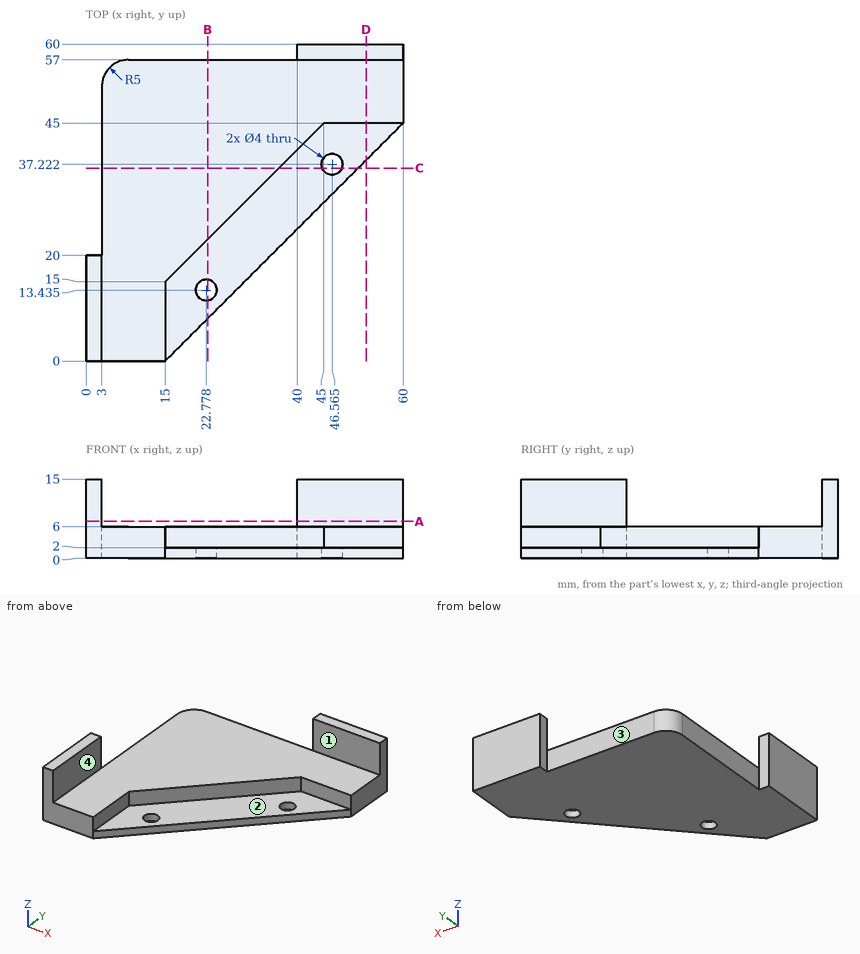
For this review, use the dimensioned drawing (mm, ordinates from the lowest corner) and the shaded views. A direction names the side the tool comes from. Round coordinates to 2 decimals unless told otherwise and drop trailing zeros. Order: outer loops, then holes, each group sorted by start corner. A loop starts at its lowest first (then second) coordinate and runs counter-clockwise, first axis right, second up. Notation, with made-up numbers: (72.5, 56.25) -> (77.5, 56.25) arc R20 ccw to (77.5, 93.25) -> close; hole circle Ø6 at (48, -19.75). An arc over 180 degrees is marked (long way). One line per item, written item: value. Start each with the question number.
Q1. Take a section at C-C (y = 36.5). Write out the cut boundary in (x, z), and give its area (3 significant figures).
Q2. Wall thickness on line 1 (Z direction, x = 14, y = 33); line 2 (Y direction, x = 55, z = 1.5); line 3 (Z direction, x = 17.5, y = 8.5): over which ranges is each line inside the solid? List them lowest first.
Q3. Take a section at D-D (x = 53). Write out the cut boundary in (y, z).
Q4. Clearance check with flat-ended pins moving along their axes: pin 1 Ø10 at (x, y) = (13.5, 27.5) entering from +Z; pin 2 Ø1.8 at (x, z) = (23.5, 2) entering from +Y; pin 3 Ø6.5 at (x, y) = (46.56, 37.22) entering from +Z; pin 4 Ø5 at (y, z) = (28.5, 10) entering from -X. State where each tip first meets the part, or that it passes through.
Q5. Take a section at A-A (z = 7). Write out the cut boundary in (x, y).
Q6. Take a section at B-B (x = 23). Write out the cut boundary in (y, z).
Q7. Machinability: for the marked faces 1, 2, 3 and 4, which of the approach directions +Z, -Z, +X, -X, +Y, -Y give a long, thin tool a straight path to every point of the face, cutting with its end or side? Answer none if there is none.
Reported:
1. outline: (3, 0) -> (44.7, 0) -> (44.7, 2) -> (36.5, 2) -> (36.5, 6) -> (3, 6) -> close; (48.43, 0) -> (51.5, 0) -> (51.5, 2) -> (48.43, 2) -> close
1. area: 224 mm2
2. line 1: z = 0 to 6
2. line 2: y = 40 to 60
2. line 3: z = 0 to 2
3. outline: (38, 0) -> (60, 0) -> (60, 15) -> (57, 15) -> (57, 6) -> (45, 6) -> (45, 2) -> (38, 2) -> close
4. pin 1: stops at z = 6
4. pin 2: stops at y = 57
4. pin 3: stops at z = 2
4. pin 4: passes through
5. outline: (0, 0) -> (3, 0) -> (3, 20) -> (0, 20) -> close; (40, 57) -> (60, 57) -> (60, 60) -> (40, 60) -> close
6. outline: (8, 0) -> (11.45, 0) -> (11.45, 2) -> (8, 2) -> close; (15.42, 0) -> (57, 0) -> (57, 6) -> (23, 6) -> (23, 2) -> (15.42, 2) -> close
7. face 1: +Z, +X, -X, -Y
7. face 2: +Z, +X, -Y
7. face 3: +Z, -Z, -X, +Y
7. face 4: +Z, +X, +Y, -Y
